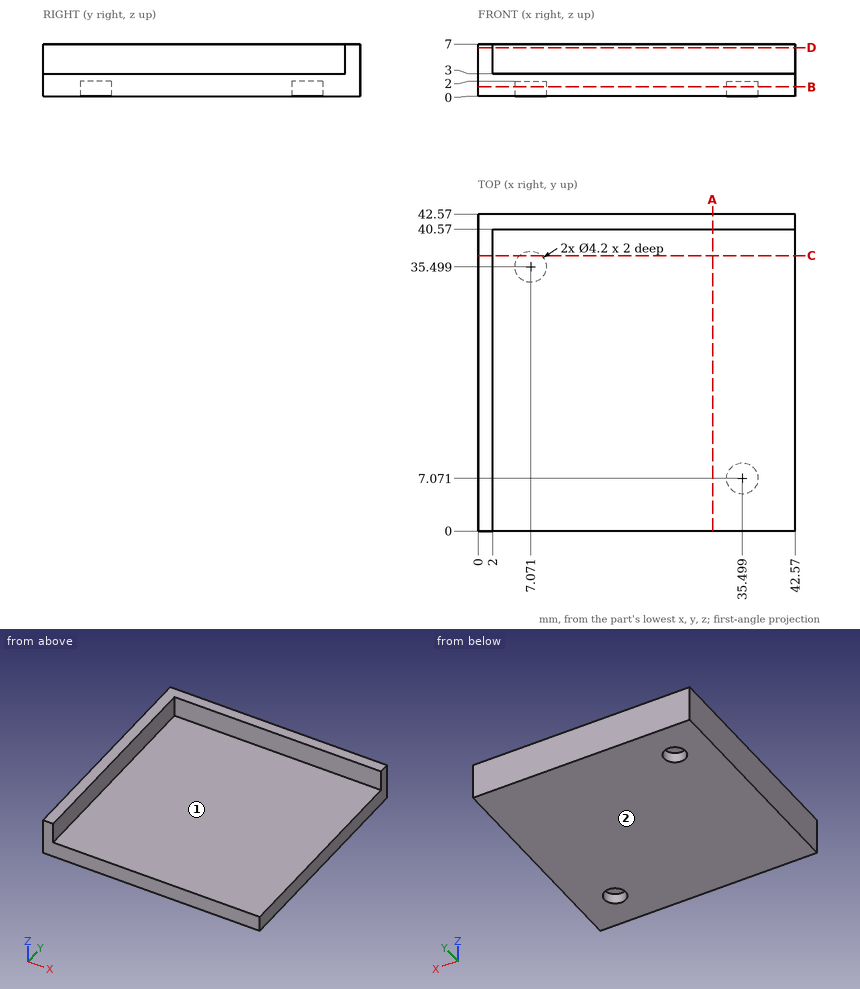
Answer from the drawing. Dimensions are ordinates in mm from the lowest x, y and z of the part. A direction names the side the tool comes from. Give positions to 0.01 mm unless a question says otherwise; leave off trailing zeros. Order: outer loops, then holes, each group sorted by start corner. A loop starts at its lowest first (then second) coordinate and runs counter-clockwise, first axis right, second up.
(1) For the marked faces 1 and 2, determine the directions among +Z, -Z, +X, -X, +Y, -Y from which every point of the face is accessible in a straight line to the end or side of a thin tool.
(2) Straight lines are drawn through the part: L1, parallel to Z at x = 18, y = 20.5; L2, parallel to Y at x = 4.5, z = 6.25; L3, parallel to X at y = 22, z = 3.75. For each, find the intervals that lie inside material, in ascending order.
(3) Given pin 1 (2 mm diameter, centred on x = 7.5, y = 36, fed in from -Z); pin 2 (10 mm diameter, centred on x = 13.5, y = 23.5, fed in from +Z); pin 3 (1.2 mm diameter, centred on y = 15, z = 6, fed in from +X), each flat-ended and moving along its own axis, determine where each tip first touches the part or whether it passes through.
(4) Find section D-D (z = 6.5). Give the vertices of the cut face in (x, y), plus the area to 3 significant figures.
(5) Find section C-C (y = 37). Give the vertices of the cut face in (x, z), plus the area to 3 significant figures.
(6) Find section A-A (x = 31.5). Give the vertices of the cut face in (y, z), plus the area to 3 significant figures.
(7) Find section B-B (z = 1.25). Give the vertices of the cut face in (x, y), plus the area to 3 significant figures.
Result sheet:
1. face 1: +Z, +X, -Y
1. face 2: -Z, +X, -X, +Y, -Y
2. L1: z = 0 to 3
2. L2: y = 40.57 to 42.57
2. L3: x = 0 to 2
3. pin 1: stops at z = 2
3. pin 2: stops at z = 3
3. pin 3: stops at x = 2
4. outline: (0, 0) - (2, 0) - (2, 40.57) - (42.57, 40.57) - (42.57, 42.57) - (0, 42.57) - close
4. area: 166 mm2
5. outline: (0, 0) - (5.6, 0) - (5.6, 2) - (8.54, 2) - (8.54, 0) - (42.57, 0) - (42.57, 3) - (2, 3) - (2, 7) - (0, 7) - close
5. area: 130 mm2
6. outline: (0, 0) - (42.57, 0) - (42.57, 7) - (40.57, 7) - (40.57, 3) - (0, 3) - close
6. area: 136 mm2
7. outline: (0, 0) - (42.57, 0) - (42.57, 42.57) - (0, 42.57) - close; hole circle Ø4.2 at (7.07, 35.5); hole circle Ø4.2 at (35.5, 7.07)
7. area: 1,780 mm2
